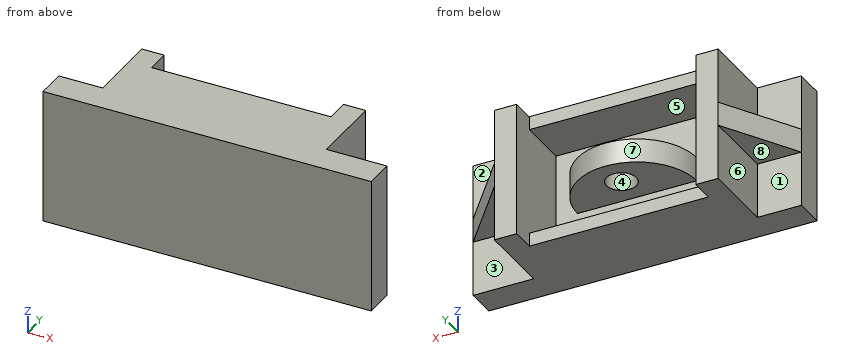
from build123d import *

# Parameters (mm, degrees)
SKETCH3_W             = 14.715370019
SKETCH3_H             = 45
BOSS_EXTRUDE4_DEPTH   = 10
SKETCH3_W_2           = 60
SKETCH3_H_2           = 36
BOSS_EXTRUDE4_2_DEPTH = 10
SKETCH3_W_3           = 20.284629981
BOSS_EXTRUDE4_3_DEPTH = 10
BOSS_EXTRUDE5_DEPTH   = 35
SKETCH3_4_W           = 60
SKETCH3_4_H           = 4.5
BOSS_EXTRUDE6_DEPTH   = 27
SKETCH4_R             = 5
BOSS_EXTRUDE7_DEPTH   = 4
RIB1_REACH            = 70.966
SKETCH5_WALL_W        = 168.940487542
SKETCH5_WALL_H        = 8
RIB2_REACH            = 70.966
SKETCH6_WALL_W        = 172.12533758
SKETCH6_WALL_H        = 8


with BuildPart() as part:
    # Sketch3 → Boss-Extrude4 (new body)
    with BuildSketch(Plane(origin=(0, 0, 0), x_dir=(1, 0, 0), z_dir=(0, 1, 0))):
        with Locations((-47.64231499, 0)):
            Rectangle(SKETCH3_W, SKETCH3_H)
    extrude(amount=BOSS_EXTRUDE4_DEPTH)



with BuildPart() as body_2:
    # Sketch3 → Boss-Extrude4 2 (new body)
    with BuildSketch(Plane(origin=(0, 0, 0), x_dir=(1, 0, 0), z_dir=(0, 1, 0))):
        with Locations((-2.784629981, 0)):
            Rectangle(SKETCH3_W_2, SKETCH3_H_2)
    extrude(amount=BOSS_EXTRUDE4_2_DEPTH)


with BuildPart() as body_3:
    # Sketch3 → Boss-Extrude4 3 (new body)
    with BuildSketch(Plane(origin=(0, 0, 0), x_dir=(1, 0, 0), z_dir=(0, 1, 0))):
        with Locations((44.85768501, 0)):
            Rectangle(SKETCH3_W_3, SKETCH3_H)
    extrude(amount=BOSS_EXTRUDE4_3_DEPTH)


with BuildPart() as part_1:
    add(part.part)

    add(body_2.part)  # Boss-Extrude5 merges body 2

    add(body_3.part)  # Boss-Extrude5 merges body 3
    # Sketch3_3 → Boss-Extrude5 (add)
    with BuildSketch(Plane(origin=(0, 0, 0), x_dir=(1, 0, 0), z_dir=(0, 1, 0))):
        Polygon((-32.784629981, 22.5), (-40.284629981, 22.5), (-40.284629981, -22.5), (-32.784629981, -22.5), (-32.784629981, -18), (-32.784629981, 18), align=None)
        Polygon((34.715370019, 22.5), (27.215370019, 22.5), (27.215370019, 18), (27.215370019, -18), (27.215370019, -22.5), (34.715370019, -22.5), align=None)
    extrude(amount=BOSS_EXTRUDE5_DEPTH)

    # Sketch3_4 → Boss-Extrude6 (add)
    with BuildSketch(Plane(origin=(0, 0, 0), x_dir=(1, 0, 0), z_dir=(0, 1, 0))):
        with Locations((-2.784629981, -20.25)):
            Rectangle(SKETCH3_4_W, SKETCH3_4_H)
        with Locations((-2.784629981, 20.25)):
            Rectangle(SKETCH3_4_W, SKETCH3_4_H)
    extrude(amount=BOSS_EXTRUDE6_DEPTH)

    # Sketch4 → Boss-Extrude7 (add, symmetric)
    with BuildSketch(Plane.XY):
        with BuildLine():
            Line((-20, 10), (20, 10))
            ThreePointArc((20, 10), (0, 30), (-20, 10))
        make_face()
        with Locations((0, 20)):
            Circle(SKETCH4_R, mode=Mode.SUBTRACT)
    extrude(amount=BOSS_EXTRUDE7_DEPTH, both=True)

    # Sketch5 wall → Rib1 (add, up to next)
    with BuildSketch(Plane(origin=(-47.64231499, 22.5, 0), x_dir=(-0.507263085957, -0.861791251769, 0), z_dir=(0.861791251769, -0.507263085957, 0)), mode=Mode.PRIVATE) as rib1_sk1:
        Rectangle(SKETCH5_WALL_W, SKETCH5_WALL_H)
    rib1_tool1 = extrude(rib1_sk1.sketch, amount=RIB1_REACH, mode=Mode.PRIVATE) - part_1.part
    add(rib1_tool1.solids().sort_by_distance((-47.64231499, 22.5, 0))[0])

    # Sketch6 wall → Rib2 (add, up to next)
    with BuildSketch(Plane(origin=(44.85768501, 22.5, 0), x_dir=(0.630071035104, -0.77653750117, 0), z_dir=(0.77653750117, 0.630071035104, 0)), mode=Mode.PRIVATE) as rib2_sk1:
        Rectangle(SKETCH6_WALL_W, SKETCH6_WALL_H)
    rib2_tool1 = extrude(rib2_sk1.sketch, amount=-RIB2_REACH, mode=Mode.PRIVATE) - part_1.part
    add(rib2_tool1.solids().sort_by_distance((44.85768501, 22.5, 0))[0])


solid = part_1.part
The listing builds one solid part. Answer for the finished solid, in the listing's coordinates (mm). Face numbers are marked on the shaded views. A direction names the side the tool comes from. Coordinates: 2 decimals unless noted, no trailing zeros. Loops run counter-clockwise (first coordinate to the right, second up) from the corner with the lowest first, then second, coordinate; pieces in that order, holes last. Notation, with made-up numbers: M 46,22 L 83,22 A20 cw 83,57 Z; hole C -26,27.25 d6. An arc over 180 degrees is marked long. Answer in a Markdown table with one row per item.
1) Find section D-D (y = 12). Determine the outline of the cut face in (x, z).
Answers below:
| item | result |
|---|---|
| outline | M -53.82,-4 L -40.28,-4 L -40.28,-22.5 L 34.72,-22.5 L 34.72,-4 L 53.38,-4 L 53.38,4 L 34.72,4 L 34.72,22.5 L -40.28,22.5 L -40.28,4 L -53.82,4 Z; M -19.9,-4 L 19.9,-4 L 19.9,4 L -19.9,4 Z; hole M -32.78,-18 L 27.22,-18 L 27.22,18 L -32.78,18 Z |
2) Find section C-C (y = 19). Determine the outline of the cut face in (x, z), then the cut area to 3 significant figures.
Answers below:
| item | result |
|---|---|
| outline | M -49.7,-4 L -40.28,-4 L -40.28,-22.5 L 34.72,-22.5 L 34.72,-4 L 47.7,-4 L 47.7,4 L 34.72,4 L 34.72,22.5 L -40.28,22.5 L -40.28,4 L -49.7,4 Z; M -17.86,-4 L -4.9,-4 L -4.9,4 L -17.86,4 Z; M 4.9,-4 L 17.86,-4 L 17.86,4 L 4.9,4 Z; hole M -32.78,-18 L 27.22,-18 L 27.22,18 L -32.78,18 Z |
| area | 1,600 mm^2 |
3) Find section B-B (z = 0). Determine the outline of the cut face in (x, y).
Answers below:
| item | result |
|---|---|
| outline | M -55,0 L 55,0 L 55,10 L 34.72,35 L 27.22,35 L 27.22,10 L 20,10 A20 ccw -20,10 L -32.78,10 L -32.78,35 L -40.28,35 L -55,10 Z; hole C 0,20 d10 |
4) Given pin 1 (12 mm diameter, centred on x = -46.5, z = 17.5, fed in from +Y); pin 2 (16 mm diameter, centred on x = 46, y = 28.5, fed in from -Z); pin 3 (5.5 mm diameter, centred on y = 23.5, z = -9.5, fed in from -X), each flat-ended and moving along its own axis, determine where each tip first touches the part or whether it passes through.
Answers below:
| item | result |
|---|---|
| pin 1 | y = 10 |
| pin 2 | z = -4 |
| pin 3 | x = -40.28 |
5) Which of the six approach directions +Z, -Z, +X, -X, +Y, -Y give full straight-line access (tool end or side, diameter ignored) to the marked faces 1, 2, 3 and 4?
Answers below:
| item | result |
|---|---|
| face 1 | -Z, -X, +Y |
| face 2 | +Z, +X, +Y |
| face 3 | -Z, +X, +Y |
| face 4 | none |
6) Determine the mould class of the marked faces 5, 6, 7 and 8 for opening direction X: released by +X, released by -X, zero draft, split by the parting line, or undercut.
Answers below:
| item | result |
|---|---|
| face 5 | undercut |
| face 6 | released by -X |
| face 7 | undercut |
| face 8 | zero draft |
7) Find the intervals of material crossed by probe 1 along Z at (x, y) = (-17, 19); probe 2 along X at (y, z) = (17, 11); probe 3 along Y at (x, z) = (0, -2.5), in increasing order.
Answers below:
| item | result |
|---|---|
| probe 1 | -22.5 to -18, -4 to 4, 18 to 22.5 |
| probe 2 | -40.28 to -32.78, 27.22 to 34.72 |
| probe 3 | 0 to 15, 25 to 30 |
8) Find section A-A (x = 0). Determine the outline of the cut face in (y, z).
Answers below:
| item | result |
|---|---|
| outline | M 0,-22.5 L 27,-22.5 L 27,-18 L 10,-18 L 10,-4 L 15,-4 L 15,4 L 10,4 L 10,18 L 27,18 L 27,22.5 L 0,22.5 Z; M 25,-4 L 30,-4 L 30,4 L 25,4 Z |
